For this review, take the finished solid that the model builds, in its own axes (mm). A direction names the side the tool comes from. Coordinates: 2 decimals unless noted, no trailing zeros. Loops run counter-clockwise (first coordinate to the right, second up) from the corner with the lowest first, then second, coordinate; pieces in that order, holes last. Notation, with made-up numbers: M 47,69.5 L 80,69.5 A10 cw 80,84.5 Z; hole C 22.5,75.25 d9. An arc over 180 degrees is marked long. Put each result on its own line as item: value.
```python
from build123d import *

# Parameters (mm, degrees)
SKETCH1_R                                     = 57.5
SKETCH1_R_2                                   = 0.5
SKETCH1_W                                     = 9.3
SKETCH1_H                                     = 9.875
BOSS_EXTRUDE1_DEPTH                           = 3
CSK_FOR_8_FLAT_HEAD_SOCKET_CAP_SCREW1_A_COUNT = 2
CSK_FOR_8_FLAT_HEAD_SOCKET_CAP_SCREW1_A_PITCH = 67.882250994
CSK_FOR_8_FLAT_HEAD_SOCKET_CAP_SCRE_2_COUNT   = 2
CSK_FOR_8_FLAT_HEAD_SOCKET_CAP_SCRE_2_PITCH   = 96
CSK_FOR_8_FLAT_HEAD_SOCKET_CAP_SCRE_3_COUNT   = 2
CSK_FOR_8_FLAT_HEAD_SOCKET_CAP_SCRE_3_PITCH   = 67.882250994
CUT_EXTRUDE1_DEPTH                            = 4
FILLET1_R                                     = 5
SKETCH5_W                                     = 4.0625
SKETCH5_H                                     = 9.875
CUT_EXTRUDE2_DEPTH                            = 4


with BuildPart() as part:
    # Sketch1 → Boss-Extrude1 (new body)
    with BuildSketch(Plane(origin=(0, 0, 0), x_dir=(1, 0, 0), z_dir=(0, 1, 0))):
        Circle(SKETCH1_R)
        with Locations((-33.941125497, 33.941125497)):
            Circle(SKETCH1_R_2, mode=Mode.SUBTRACT)
        with Locations((33.941125497, 33.941125497)):
            Circle(SKETCH1_R_2, mode=Mode.SUBTRACT)
        with Locations((33.941125497, -33.941125497)):
            Circle(SKETCH1_R_2, mode=Mode.SUBTRACT)
        with Locations((-33.941125497, -33.941125497)):
            Circle(SKETCH1_R_2, mode=Mode.SUBTRACT)
        with Locations((1.65, 0)):
            Rectangle(SKETCH1_W, SKETCH1_H, mode=Mode.SUBTRACT)
    extrude(amount=BOSS_EXTRUDE1_DEPTH)

    # Sketch2 → CSK for #8 Flat Head Socket Cap Screw1 (revolve, cut)
    with BuildSketch(Plane(origin=(-33.941125497, 0, 33.941125497), x_dir=(0, 0, -1), z_dir=(1, 0, 0))):
        Polygon((0, 0), (0, 3), (2.45745, 3), (2.45745, 2.417901837), (4.5593, 0), align=None)
    csk_for_8_flat_head_socket_cap_screw1 = revolve(axis=Axis((-33.941125497, -6.35, 33.941125497), (0, 1, 0)), mode=Mode.SUBTRACT)

    # CSK for #8 Flat Head Socket Cap Screw1 a: CSK for #8 Flat Head Socket Cap Screw1 ×2
    with Locations(*[(i * CSK_FOR_8_FLAT_HEAD_SOCKET_CAP_SCREW1_A_PITCH, 0, 0) for i in range(1, CSK_FOR_8_FLAT_HEAD_SOCKET_CAP_SCREW1_A_COUNT)]):
        add(csk_for_8_flat_head_socket_cap_screw1, mode=Mode.SUBTRACT)

    # CSK for _8 Flat Head Socket Cap Scre 2: CSK for #8 Flat Head Socket Cap Screw1 ×2
    with Locations(*[Vector(0.707106781, 0, -0.707106781) * (i * CSK_FOR_8_FLAT_HEAD_SOCKET_CAP_SCRE_2_PITCH) for i in range(1, CSK_FOR_8_FLAT_HEAD_SOCKET_CAP_SCRE_2_COUNT)]):
        add(csk_for_8_flat_head_socket_cap_screw1, mode=Mode.SUBTRACT)

    # CSK for _8 Flat Head Socket Cap Scre 3: CSK for #8 Flat Head Socket Cap Screw1 ×2
    with Locations(*[(0, 0, -i * CSK_FOR_8_FLAT_HEAD_SOCKET_CAP_SCRE_3_PITCH) for i in range(1, CSK_FOR_8_FLAT_HEAD_SOCKET_CAP_SCRE_3_COUNT)]):
        add(csk_for_8_flat_head_socket_cap_screw1, mode=Mode.SUBTRACT)

    # Sketch4 → Cut-Extrude1 (cut, through all)
    with BuildSketch(Plane(origin=(0, 3, 0), x_dir=(1, 0, 0), z_dir=(0, 1, 0))):
        with BuildLine():
            Line((-26.975205126, 39.703127187), (-4.658742812, 17.386664873))
            ThreePointArc((-4.658742812, 17.386664873), (0, 18), (4.658742812, 17.386664873))
            Line((4.658742812, 17.386664873), (26.975205126, 39.703127187))
            ThreePointArc((26.975205126, 39.703127187), (0, 48), (-26.975205126, 39.703127187))
        make_face()
        with BuildLine():
            Line((39.703127187, 26.975205126), (17.386664873, 4.658742812))
            ThreePointArc((17.386664873, 4.658742812), (18, 0), (17.386664873, -4.658742812))
            Line((17.386664873, -4.658742812), (39.703127187, -26.975205126))
            ThreePointArc((39.703127187, -26.975205126), (48, 0), (39.703127187, 26.975205126))
        make_face()
        with BuildLine():
            Line((26.975205126, -39.703127187), (4.658742812, -17.386664873))
            ThreePointArc((4.658742812, -17.386664873), (0, -18), (-4.658742812, -17.386664873))
            Line((-4.658742812, -17.386664873), (-26.975205126, -39.703127187))
            ThreePointArc((-26.975205126, -39.703127187), (0, -48), (26.975205126, -39.703127187))
        make_face()
        with BuildLine():
            Line((-39.703127187, -26.975205126), (-17.386664873, -4.658742812))
            ThreePointArc((-17.386664873, -4.658742812), (-18, 0), (-17.386664873, 4.658742812))
            Line((-17.386664873, 4.658742812), (-39.703127187, 26.975205126))
            ThreePointArc((-39.703127187, 26.975205126), (-48, 0), (-39.703127187, -26.975205126))
        make_face()
    extrude(amount=-CUT_EXTRUDE1_DEPTH, mode=Mode.SUBTRACT)

    # Fillet1
    fillet1_edges = [part.edges().sort_by_distance(p)[0] for p in [
        (-39.703127187, 1.5, 26.975205126),
        (-39.703127187, 1.5, -26.975205126),
        (-26.975205126, 1.5, -39.703127187),
        (26.975205126, 1.5, -39.703127187),
        (39.703127187, 1.5, -26.975205126),
        (26.975205126, 1.5, 39.703127187),
        (-26.975205126, 1.5, 39.703127187),
    ]]
    fillet(fillet1_edges, radius=FILLET1_R)

    # Sketch5 → Cut-Extrude2 (cut, through all)
    with BuildSketch(Plane.XZ):
        with Locations((8.33125, 0)):
            Rectangle(SKETCH5_W, SKETCH5_H)
        with Locations((-5.03125, 0)):
            Rectangle(SKETCH5_W, SKETCH5_H)
    extrude(amount=-CUT_EXTRUDE2_DEPTH, mode=Mode.SUBTRACT)


solid = part.part
```
(1) Add section B-B (z = 0). Write out the cut boundary in (x, y), plus the area to 3 significant figures.
Determined:
outline: M -57.5,0 L -48,0 L -48,3 L -57.5,3 Z; M -18,0 L -7.06,0 L -7.06,3 L -18,3 Z; M 10.36,0 L 18,0 L 18,3 L 10.36,3 Z; M 48,0 L 57.5,0 L 57.5,3 L 48,3 Z
area: 113 mm^2
(2) For pin 1 (1.5 mm diameter, centred on x = -23, y = 2, fed in from +Z); pin 2 (1 mm diameter, centred on x = 44, z = -24, fed in from -Y); pin 3 (1 mm diameter, centred on y = 1, z = 10, fed in from -X); pin 4 (0.9 mm diameter, centred on y = 1, z = -1, fed in from +X), all flat-tipped, find the tip position at first contact; note any pin that passes through.
Determined:
pin 1: stops at z = 53.02
pin 2: stops at y = 0
pin 3: stops at x = -56.71
pin 4: stops at x = 57.5
(3) Draft analysis for pull direction X (two halves, no side actions). For faces 3 (the cylindrical face through (39.41, 1.48, -23.79)), 4 (the flat face through (-1, 3, 12)), 5 (the cylindrical face through (-12.465, 1.479, 56.133)), state which applies: +X half, -X half, draft (parallel to the pull), parting line (faces both ways), or undercut.
Determined:
face 3: undercut
face 4: draft
face 5: parting line
(4) Add section C-C (x = 13.5). Write out the cut boundary in (y, z), plus the area to 3 significant figures.
Determined:
outline: M 0,-55.89 L 3,-55.89 L 3,-46.06 L 0,-46.06 Z; M 0,-26.23 L 3,-26.23 L 3,26.23 L 0,26.23 Z; M 0,46.06 L 3,46.06 L 3,55.89 L 0,55.89 Z
area: 216 mm^2
(5) Wall thickness on line 1 along X through (y, z) = (2.9, 0.5); line 2 along Z through (x, y) = (14.5, 1.8); line 3 along X through (y, z) = (0.4, 34): over which ranges is each line inside the solid? List them lowest first. Write a range as [from, to].
Determined:
line 1: x = [-57.5, -48], [-17.99, -7.06], [10.36, 17.99], [48, 57.5]
line 2: z = [-55.64, -45.76], [-27.23, 27.23], [45.76, 55.64]
line 3: x = [-46.37, -38.15], [-29.73, -21.27], [21.27, 29.73], [38.15, 46.37]
(6) Add section A-A (x = 0). Write out the cut boundary in (y, z), plus the area to 3 significant figures.
Determined:
outline: M 0,-57.5 L 3,-57.5 L 3,-48 L 0,-48 Z; M 0,-18 L 3,-18 L 3,-4.94 L 0,-4.94 Z; M 0,4.94 L 3,4.94 L 3,18 L 0,18 Z; M 0,48 L 3,48 L 3,57.5 L 0,57.5 Z
area: 135 mm^2
(7) Add section D-D (y = 1.6). State how many separate pieces and enclosed holes the cut face has, plus the area to 3 significant figures.
Determined:
separate pieces: 1
enclosed holes: 9
area: 6,130 mm^2
(8) Tool access review of faces 1 (the flat face through (-1, 0, 12)), 2 (the flat face through (-26.13, 1.52, -13.4)): name each direction out of +Z, -Z, +X, -X, +Y, -Y from which nothing blocks a thin tool from reaching the whole face with its end or side.
Determined:
face 1: +Z, -Z, +X, -X, -Y
face 2: +Y, -Y
